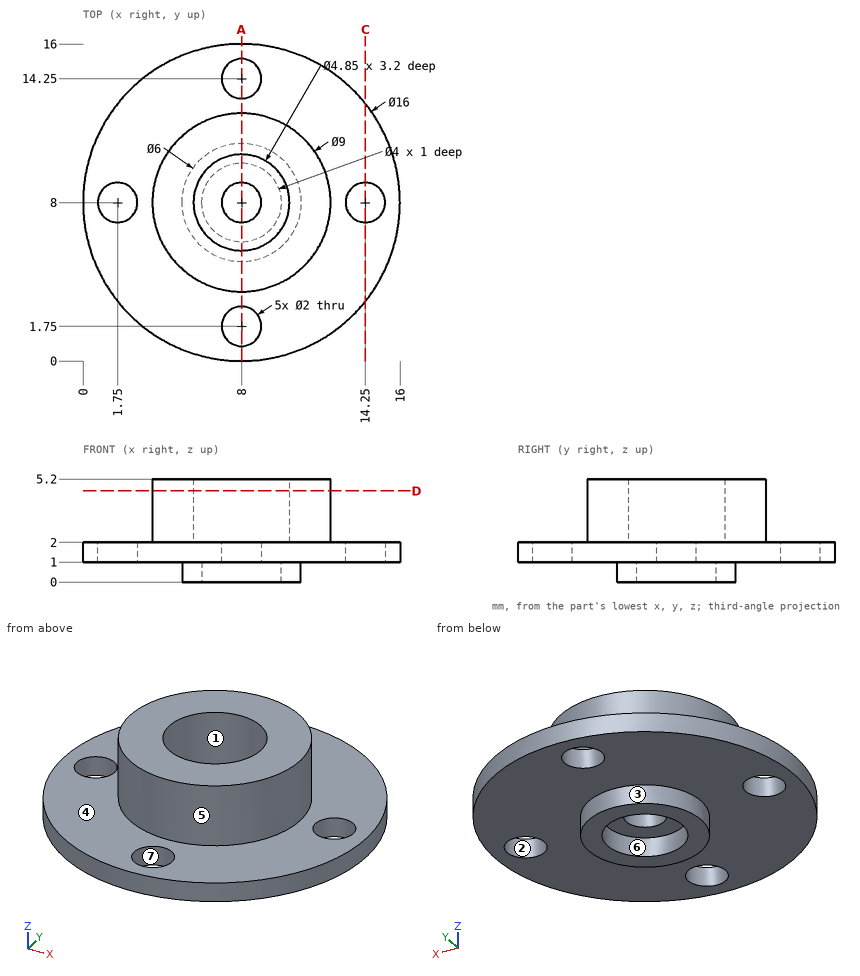
Print and shaded views of the part. All mm, measured from the part's lowest x, y and z. A direction names the side the tool comes from. Coordinates: 2 decimals unless noted, no trailing zeros. Order: outer loops, then holes, each group sorted by start corner. A loop starts at its lowest first (then second) coordinate and runs counter-clockwise, first axis right, second up. Notation, with made-up numbers: (89.5, 44.5) -> (145.5, 44.5) arc R17 cw to (145.5, 71.5) -> close; hole circle Ø7 at (16.5, -12.75). An arc over 180 degrees is marked (long way). Use one line per item in the form item = value. Start each with the question number.
1) Pull direction Y, two halves, no side cores. Call the marked faces 4, 5, 6 and 7: +Y half, -Y half, draft (parallel to the pull), parting line (faces both ways), or undercut.
2) Band-saw the part on D-D on z = 4.6. Give the cut face in (x, y) (3 decimals).
3) Drop flat-ended pins along their axis: pin 1 (3 mm diameter, centred on x = 7.5, z = 4.5, fed in from -Y); pin 2 (2.5 mm diameter, centred on x = 8, y = 14.25, fed in from +Z); pin 3 (3 mm diameter, centred on x = 8, y = 8, fed in from -Z). Give the stop position or say it passes through.
4) Tool access for the marked faces 1, 2 and 3: list every direction of +Z, -Z, +X, -X, +Y, -Y with a clear straight run to the whole face (end or side of a thin tool).
5) Band-saw the part on C-C on x = 14.25. Give the cut face in (y, z), then the cut area to 3 significant figures.
6) Drill centre lines: L1, parallel to Y at x = 8, z = 1.4; L2, parallel to Z at x = 10.75, y = 14.75; L3, parallel to Y at x = 9.75, z = 3.1. Where is each one in solid material? Low to high. Write a range as [from, to].
7) Band-saw the part on A-A on x = 8. State how many separate pieces and enclosed holes the cut face has, then the cut area to 3 significant figures.
Entries:
q1.face_4 = draft
q1.face_5 = parting line
q1.face_6 = undercut
q1.face_7 = undercut
q2.outline = circle Ø9 at (8, 8); hole circle Ø4.85 at (8, 8)
q3.pin_1 = 3.5
q3.pin_2 = 2
q3.pin_3 = 1
q4.face_1 = +Z
q4.face_2 = +Z, -Z
q4.face_3 = -Z
q5.outline = (3.01, 1) -> (7, 1) -> (7, 2) -> (3.01, 2) -> close; (9, 1) -> (12.99, 1) -> (12.99, 2) -> (9, 2) -> close
q5.area = 7.99 mm2
q6.L1 = [0, 0.75], [2.75, 7], [9, 13.25], [15.25, 16]
q6.L2 = [1, 2]
q6.L3 = [3.85, 6.32], [9.68, 12.15]
q7.separate_pieces = 4
q7.enclosed_holes = 0
q7.area = 25.3 mm2
